Part model, mm, in its own coordinate system. Face numbers are marked on the shaded views. A direction names the side the tool comes from. Round coordinates to 2 decimals unless told otherwise and drop trailing zeros. Loops run counter-clockwise (first coordinate to the right, second up) from the corner with the lowest first, then second, coordinate; pieces in that order, holes last. Notation, with made-up numbers: M 34.25,-32.5 L 55.25,-32.5 A22 ccw 55.25,-9.5 Z; hole C -35.5,78.25 d2. An arc over 180 degrees is marked long. Put each result on its own line as item: value. Start each with the question number.
1) Probe line 1 along Z through (x, y) = (5, 1); line 2 along X through (y, z) = (2.65, -83); line 3 along Y through (x, z) = (15, -43). List the from-to ranges inside material, lowest first.
2) Slice it at C-C on z = -121. Give the cut face in (x, y).
3) Slice it at A-A on z = -22. Give the cut face in (x, y).
4) Slice it at B-B on x = 5. Give the cut face in (y, z).
5) Pull direction Z, two halves, no side cores. Call the marked faces 3 and 4: +Z half, -Z half, draft (parallel to the pull), parting line (faces both ways), or undercut.
6) Slice it at D-D on x = 51.5. Give the cut face in (y, z).
7) Drop flat-ended pins along their axis: pin 1 Ø3.5 at (x, z) = (30, -123.5) entering from +Y; pin 2 Ø6 at (x, z) = (18.5, -64.5) entering from +Y. Give the stop position or say it passes through.
8) Which spindle directions (+Z, -Z, +X, -X, +Y, -Y) get a long thin tool onto all of the face, cutting with end or side? Do the marked faces 1 and 2. Say none if no direction does.
```python
from build123d import *

# Parameters (mm, degrees)
SKETCH1_W               = 60
SKETCH1_H               = 130
BOSS_EXTRUDE1_DEPTH     = 1.57
SKETCH2_W               = 14.34441586
SKETCH2_H               = 47.463140714
BOSS_EXTRUDE2_DEPTH     = 3
BOSS_EXTRUDE6_START     = -1.57
BOSS_EXTRUDE6_OUTLINE_R = 2
BOSS_EXTRUDE6_DEPTH     = 1.57
SKETCH4_R               = 6
BOSS_EXTRUDE7_DEPTH     = 0.1
SKETCH5_W               = 13.72
SKETCH5_H               = 14.56
SKETCH5_H_2             = 14.76
BOSS_EXTRUDE8_DEPTH     = 0.1
SKETCH6_W               = 6.4
SKETCH6_H               = 13.8
BOSS_EXTRUDE9_DEPTH     = 0.1
SKETCH7_W               = 6.7
SKETCH7_H               = 7.7
BOSS_EXTRUDE10_DEPTH    = 0.1


# Read off the part's stored shape, not the designer's step: Boss-Extrude6
with BuildPart() as part:
    # Sketch1 → Boss-Extrude1 (new body)
    with BuildSketch(Plane(origin=(0, 0, 0), x_dir=(1, 0, 0), z_dir=(0, 1, 0))):
        with Locations((30, 65)):
            Rectangle(SKETCH1_W, SKETCH1_H)
    extrude(amount=BOSS_EXTRUDE1_DEPTH)

    # Sketch2 → Boss-Extrude2 (add)
    with BuildSketch(Plane(origin=(0, 1.57, 0), x_dir=(-1, 0, 0), z_dir=(0, 1, 0))):
        with Locations((-31.510634486, -64.593919343)):
            Rectangle(SKETCH2_W, SKETCH2_H)
    extrude(amount=BOSS_EXTRUDE2_DEPTH)

    # Boss-Extrude6 outline → Boss-Extrude6 (cut)
    with BuildSketch(Plane(origin=(0, 1.57, 0), x_dir=(-1, 0, 0), z_dir=(0, 1, 0)).offset(BOSS_EXTRUDE6_START)):
        with Locations((-5, -5)):
            Circle(BOSS_EXTRUDE6_OUTLINE_R)
        with Locations((-55, -22)):
            Circle(BOSS_EXTRUDE6_OUTLINE_R)
        with Locations((-5, -125)):
            Circle(BOSS_EXTRUDE6_OUTLINE_R)
        with Locations((-55, -108)):
            Circle(BOSS_EXTRUDE6_OUTLINE_R)
    extrude(amount=BOSS_EXTRUDE6_DEPTH, mode=Mode.SUBTRACT)

    # Sketch4 → Boss-Extrude7 (add)
    with BuildSketch(Plane(origin=(0, 1.57, 0), x_dir=(-1, 0, 0), z_dir=(0, 1, 0))):
        with Locations(Location((-32.5, -8.5, 0), (0, 0, 270))):
            Circle(SKETCH4_R)
        with Locations(Location((-51.5, -8.5, 0), (0, 0, 270))):
            Circle(SKETCH4_R)
        with Locations(Location((-32.5, -121, 0), (0, 0, 270))):
            Circle(SKETCH4_R)
        with Locations(Location((-51.5, -121, 0), (0, 0, 270))):
            Circle(SKETCH4_R)
    extrude(amount=BOSS_EXTRUDE7_DEPTH)

    # Sketch5 → Boss-Extrude8 (add)
    with BuildSketch(Plane(origin=(0, 1.57, 0), x_dir=(-1, 0, 0), z_dir=(0, 1, 0))):
        with Locations((-8.36, -20)):
            Rectangle(SKETCH5_W, SKETCH5_H)
        with Locations((-8.36, -39)):
            Rectangle(SKETCH5_W, SKETCH5_H_2)
    extrude(amount=BOSS_EXTRUDE8_DEPTH)

    # Sketch6 → Boss-Extrude9 (add)
    with BuildSketch(Plane(origin=(2.04497346, 1.57, -23.026190138), x_dir=(-1, 0, 0), z_dir=(0, 1, 0))):
        with Locations((-3.3, -86.9)):
            Rectangle(SKETCH6_W, SKETCH6_H)
    extrude(amount=BOSS_EXTRUDE9_DEPTH)

    # Sketch7 → Boss-Extrude10 (add)
    with BuildSketch(Plane(origin=(0.458943498, 1.57, 31.036587212), x_dir=(-1, 0, 0), z_dir=(0, 1, 0))):
        with Locations((-3.45, -103.85)):
            Rectangle(SKETCH7_W, SKETCH7_H)
    extrude(amount=BOSS_EXTRUDE10_DEPTH)


solid = part.part
```
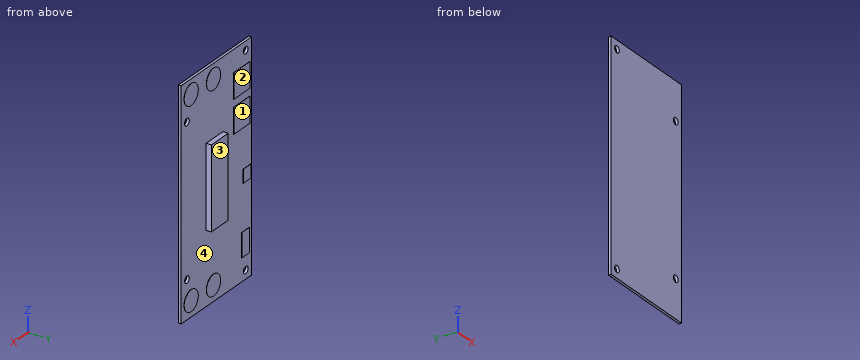
Recorded:
1. line 1: z = -130 to -127, -123 to -7, -3 to 0
1. line 2: x = 24.34 to 38.68
1. line 3: y = 0 to 1.67
2. outline: M 0,0 L 60,0 L 60,1.57 L 57.5,1.57 L 57.5,1.67 L 45.5,1.67 L 45.5,1.57 L 38.5,1.57 L 38.5,1.67 L 26.5,1.67 L 26.5,1.57 L 0,1.57 Z
3. outline: M 0,0 L 53,0 L 53,1.57 L 15.22,1.57 L 15.22,1.67 L 1.5,1.67 L 1.5,1.57 L 0,1.57 Z; M 57,0 L 60,0 L 60,1.57 L 57,1.57 Z
4. outline: M 0,-130 L 1.57,-130 L 1.57,-127 L 0,-127 Z; M 0,-123 L 1.57,-123 L 1.57,-116.83 L 1.67,-116.83 L 1.67,-103.03 L 1.57,-103.03 L 1.57,-76.66 L 1.67,-76.66 L 1.67,-68.96 L 1.57,-68.96 L 1.57,-46.38 L 1.67,-46.38 L 1.67,-31.62 L 1.57,-31.62 L 1.57,-27.28 L 1.67,-27.28 L 1.67,-12.72 L 1.57,-12.72 L 1.57,-7 L 0,-7 Z; M 0,-3 L 1.57,-3 L 1.57,0 L 0,0 Z
5. face 3: draft
5. face 4: undercut
6. outline: M 0,-130 L 1.57,-130 L 1.57,-127 L 1.67,-127 L 1.67,-115 L 1.57,-115 L 1.57,-14.5 L 1.67,-14.5 L 1.67,-2.5 L 1.57,-2.5 L 1.57,0 L 0,0 Z
7. pin 1: stops at y = 1.67
7. pin 2: stops at y = 1.57
8. face 1: +Z, -Z, -X, +Y
8. face 2: +Z, -Z, +X, -X, +Y
